from build123d import *

# Parameters (mm, degrees)
EXTRUDE_1_DEPTH          = 35
SKETCH_2_W               = 110
SKETCH_2_H               = 45
EXTRUDE_2_DEPTH          = 10
CUT_EXTRUDE_1_DEPTH      = 85.198125322
CUT_EXTRUDE_1_DEPTH_BACK = 85.198125322
CUT_EXTRUDE_2_DEPTH      = 50
FILLET_2_R               = 15


with BuildPart() as part:
    # 스케치1 → 보스-돌출1 (new body)
    with BuildSketch(Plane.XY):
        Polygon((-55, 0), (55, 0), (55, 10), (27, 10), (27, 45.158878505), (-27, 45.158878505), (-27, 10), (-55, 10), align=None)
    extrude(amount=EXTRUDE_1_DEPTH)

    # 스케치2 → 보스-돌출2 (add)
    with BuildSketch(Plane(origin=(0, 0, 0), x_dir=(-1, 0, 0), z_dir=(0, 0, -1))):
        with Locations((0, 22.5)):
            Rectangle(SKETCH_2_W, SKETCH_2_H)
    extrude(amount=EXTRUDE_2_DEPTH)

    # 스케치3 → 컷-돌출1 (cut, two sides: drawn at the far end of the back side and taken through both)
    with BuildSketch(Plane.XY.offset(35).offset(-CUT_EXTRUDE_1_DEPTH_BACK)):
        with BuildLine():
            ThreePointArc((-16, 45.158878505), (0, 29.158878505), (16, 45.158878505))
            Line((16, 45.158878505), (-16, 45.158878505))
        make_face()
    extrude(amount=CUT_EXTRUDE_1_DEPTH + CUT_EXTRUDE_1_DEPTH_BACK, mode=Mode.SUBTRACT)

    # 스케치4 → 컷-돌출2 (cut)
    with BuildSketch(Plane(origin=(0, 0, -10), x_dir=(-1, 0, 0), z_dir=(0, 0, -1))):
        with BuildLine():
            Line((-19, 45.158878505), (19, 45.158878505))
            ThreePointArc((19, 45.158878505), (0, 26.158878505), (-19, 45.158878505))
        make_face()
    extrude(amount=-CUT_EXTRUDE_2_DEPTH, mode=Mode.SUBTRACT)

    # 스케치12 → M8 소켓 머리 캡 나사용 카운터보어5 (revolve, cut)
    with BuildSketch(Plane(origin=(-40, 38.932438824, 0), x_dir=(0, -1, 0), z_dir=(1, 0, 0))):
        Polygon((0, 0), (0, 10), (4.5, 10), (4.5, 8), (7, 8), (7, 0.024142219), (7.025, 0), align=None)
    revolve(axis=Axis((-40, 38.932438824, 6.35), (0, 0, -1)), mode=Mode.SUBTRACT)

    # 스케치13 → M8 소켓 머리 캡 나사용 카운터보어4 (revolve, cut)
    with BuildSketch(Plane(origin=(-46.472033472, 10, 20), x_dir=(0, 0, 1), z_dir=(1, 0, 0))):
        Polygon((0, 0), (0, 10), (4.5, 10), (4.5, 8), (7, 8), (7, 0.024142219), (7.025, 0), align=None)
    revolve(axis=Axis((-46.472033472, 16.35, 20), (0, -1, 0)), mode=Mode.SUBTRACT)

    # 스케치15 → M8 소켓 머리 캡 나사용 카운터보어3 (revolve, cut)
    with BuildSketch(Plane(origin=(45.201027452, 10, 20), x_dir=(0, 0, 1), z_dir=(1, 0, 0))):
        Polygon((0, 0), (0, 10), (4.5, 10), (4.5, 8), (7, 8), (7, 0.024142219), (7.025, 0), align=None)
    revolve(axis=Axis((45.201027452, 16.35, 20), (0, -1, 0)), mode=Mode.SUBTRACT)

    # 스케치16 → M8 소켓 머리 캡 나사용 카운터보어6 (revolve, cut)
    with BuildSketch(Plane(origin=(40, 38.932438824, 0), x_dir=(0, -1, 0), z_dir=(1, 0, 0))):
        Polygon((0, 0), (0, 10), (4.5, 10), (4.5, 8), (7, 8), (7, 0.024142219), (7.025, 0), align=None)
    revolve(axis=Axis((40, 38.932438824, 6.35), (0, 0, -1)), mode=Mode.SUBTRACT)

    # 필렛2
    fillet_2_edges = [part.edges().sort_by_distance(p)[0] for p in [
        (-55, 45, -5),
        (55, 45, -5),
        (55, 5, 35),
        (-55, 5, 35),
    ]]
    fillet(fillet_2_edges, radius=FILLET_2_R)


solid = part.part
Geometry check sheet. Reference: the model listing, model coordinates, mm. A direction names the side the tool comes from. Round coordinates to 2 decimals unless told otherwise and drop trailing zeros. Order: outer loops, then holes, each group sorted by start corner. A loop starts at its lowest first (then second) coordinate and runs counter-clockwise, first axis right, second up. Notation, with made-up numbers: (86.5, 51.5) -> (108.5, 51.5) arc R21 cw to (108.5, 90.5) -> close; hole circle Ø9 at (3.25, 53). An arc over 180 degrees is marked (long way). Use one line per item in the form item = value.
1. Cross-section at A-A, the plane z = 10. Enter the section's corners in (x, y).
Working result:
outline = (-55, 0) -> (55, 0) -> (55, 10) -> (27, 10) -> (27, 45.16) -> (19, 45.16) arc R19 cw to (-19, 45.16) -> (-27, 45.16) -> (-27, 10) -> (-55, 10) -> close
2. Set-up check for faces 5 (the face through (-27, 28, 17)), 6 (the face through (27, 45, -5)), 7 (the face through (-39.156, 31.984, -3.956)), 8 (the face through (27, 27, 17)): record each of +Z, -Z, +X, -X, +Y, -Y from which the full face is reachable in a straight line by a thin tool's end or side.
Working result:
face_5 = +Z, -X, +Y
face_6 = -Z, +X, -X, +Y
face_7 = +Z
face_8 = +Z, +X, +Y
3. Scan lines: line 1 along Y through (x, z) = (40, -9); line 2 along X through (y, z) = (7, 14.5); line 3 along Y through (x, z) = (-31, -6). Record each from-to range of solid material in increasing order. Write a range as from..to.
Working result:
line_1 = 0..34.43, 43.43..45
line_2 = -55..-50.8, -42.14..40.87, 49.53..55
line_3 = 0..45
4. Cross-section at C-C, the plane y = 22. Enter the section's corners in (x, z).
Working result:
outline = (-55, -10) -> (55, -10) -> (55, 0) -> (27, 0) -> (27, 35) -> (-27, 35) -> (-27, 0) -> (-55, 0) -> close
5. Cross-section at B-B, the plane y = 6.5. Enter the section's corners in (x, z).
Working result:
outline = (-55, -10) -> (55, -10) -> (55, 20) arc R15 ccw to (40, 35) -> (-40, 35) arc R15 ccw to (-55, 20) -> close; hole circle Ø14 at (-46.47, 20); hole circle Ø14 at (45.2, 20)
6. Go/stop test with flat-tipped pins: pin 1 (12.5 mm diameter, centred on x = 45.2, z = 20, fed in from +Y); pin 2 (14.5 mm diameter, centred on x = -46.47, z = 20, fed in from +Y); pin 3 (10.5 mm diameter, centred on x = 37, y = 35.5, fed in from +Z). Record where each tip stops, or that it passes through.
Working result:
pin_1 = 2
pin_2 = 10
pin_3 = 0
7. Cross-section at D-D, the plane x = 0. Enter the section's corners in (y, z).
Working result:
outline = (0, -10) -> (26.16, -10) -> (26.16, 35) -> (0, 35) -> close
8. Mould release check, pull along Z, two halves, no side actions. Record for faces 1 (the face through (50.72, 5.07, 30.49)), 2 (the face through (50, 2, 20)), 3 (the face through (-36.008, 36.856, -8.986)), 4 (the face through (-42.213, 6.044, 14.445)): pulls with the +Z half, pulls with the -Z half, needs draft (parallel to the pull), parting line crosses it, or undercut.
Working result:
face_1 = pulls with the +Z half
face_2 = undercut
face_3 = needs draft
face_4 = undercut
